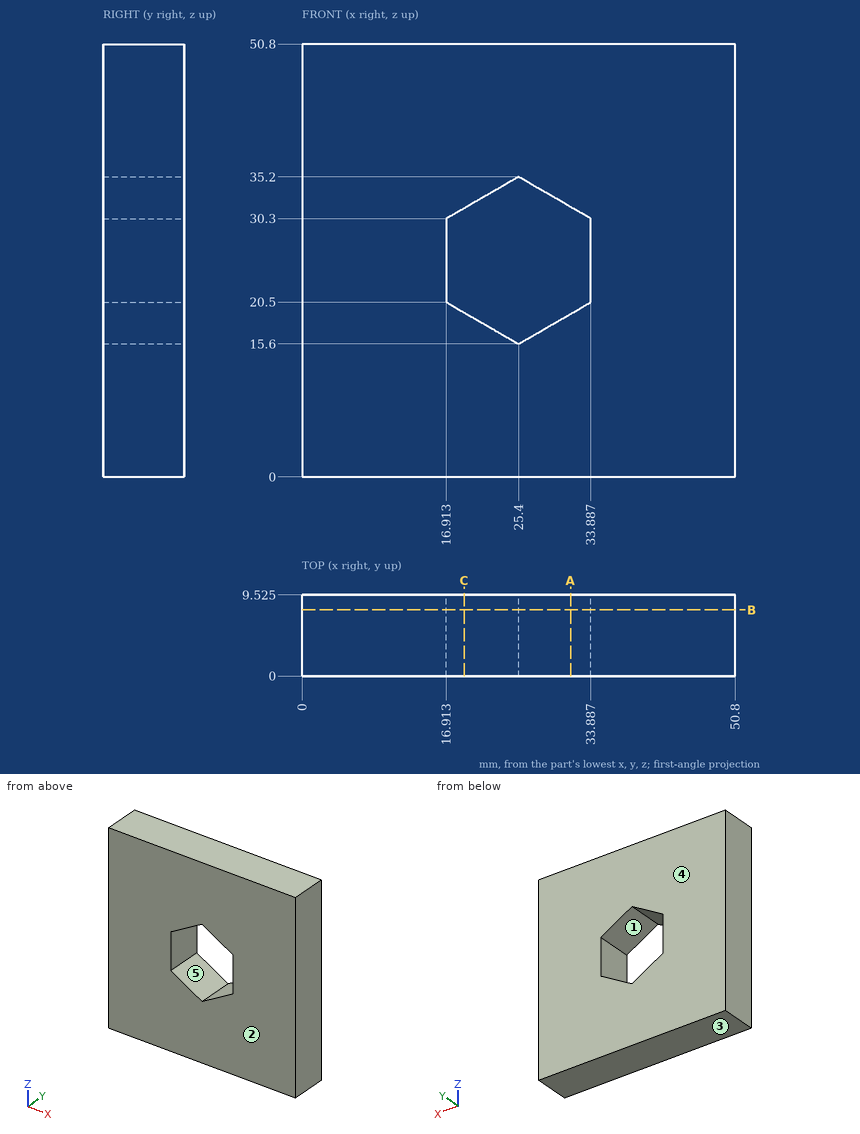
Can you work these out from the drawing? Everything is in mm from the part's minimum corner. A direction names the side the tool comes from. Round coordinates to 2 decimals unless told otherwise and drop trailing zeros. Loops run counter-clockwise (first coordinate to the right, second up) from the corner with the lowest first, then second, coordinate; pieces in that order, holes last. Notation, with made-up numbers: (55, 12.5) - (94, 12.5) arc R17 ccw to (94, 31.5) - close; hole circle Ø8 at (-15, 18). An arc over 180 degrees is marked (long way). Answer as CSV lines item,"result".
1. Please list where these lines run through material, in increasing order: line 1 along X through (y, z) = (1, 21.5); line 2 along Z through (x, y) = (21, 0.5); line 3 along X through (y, z) = (8.5, 18). Write a range as [from, to].
Filled in:
line 1,"x = [0, 16.91], [33.89, 50.8]"
line 2,"z = [0, 18.14], [32.66, 50.8]"
line 3,"x = [0, 21.24], [29.56, 50.8]"
2. On a 3-axis mill with a long thin cutter (end or side, diameter ignored), from which of +Z, -Z, +X, -X, +Y, -Y can I reach the whole of each face in a straight line? I mean the marked faces 4 and 5. Say none if no direction works.
Filled in:
face 4,"+Z, -Z, +X, -X, +Y"
face 5,"+Y, -Y"
3. We'd pull the mould along Z, two halves only. Please class the marked faces 1, 2 and 3: +Z half, -Z half, draft (parallel to the pull), parting line (faces both ways), or undercut.
Filled in:
face 1,"undercut"
face 2,"draft"
face 3,"-Z half"
4. I want a section at A-A on x = 31.5. List the corners of the cut face in (y, z) for me (3 decimals), then the cut area to 3 significant figures.
Filled in:
outline,"(0, 0) - (9.525, 0) - (9.525, 19.122) - (0, 19.122) - close; (0, 31.678) - (9.525, 31.678) - (9.525, 50.8) - (0, 50.8) - close"
area,"364 mm^2"
5. I want a section at B-B on y = 7.75. List the corners of the cut face in (x, z) for me.
Filled in:
outline,"(0, 0) - (50.8, 0) - (50.8, 50.8) - (0, 50.8) - close; hole (16.91, 20.5) - (25.4, 15.6) - (33.89, 20.5) - (33.89, 30.3) - (25.4, 35.2) - (16.91, 30.3) - close"
6. I want a section at C-C on x = 19. List the corners of the cut face in (y, z) for me (3 decimals).
Filled in:
outline,"(0, 0) - (9.525, 0) - (9.525, 19.295) - (0, 19.295) - close; (0, 31.505) - (9.525, 31.505) - (9.525, 50.8) - (0, 50.8) - close"
